Model file for the job. Use its own axes, mm. A direction names the side the tool comes from. Coordinates: 2 decimals unless noted, no trailing zeros. Write each loop counter-clockwise with the first axis right and the second up, starting at its lowest first coordinate (ties: lowest second). Pieces come first, ordered by that corner, then holes. Notation, with made-up numbers: (2.25, 48) -> (60.25, 48) arc R15 ccw to (60.25, 75) -> close; hole circle Ø5 at (81, 55). An arc over 180 degrees is marked (long way). Write item = value, one per line. Start each with the question number.
from build123d import *

# Parameters (mm, degrees)
SKETCH1_R           = 6
BOSS_EXTRUDE1_DEPTH = 4
SKETCH2_R           = 3
BOSS_EXTRUDE2_DEPTH = 4
SKETCH3_R           = 1.6
CUT_EXTRUDE1_DEPTH  = 16
CHAMFER1_SIZE       = 3


with BuildPart() as part:
    # Sketch1 → Boss-Extrude1 (new, symmetric)
    with BuildSketch(Plane(origin=(0, 0, 0), x_dir=(1, 0, 0), z_dir=(0, 1, 0))):
        with Locations(Location((0, 0, 0), (0, 0, 270))):
            Circle(SKETCH1_R)
    extrude(amount=BOSS_EXTRUDE1_DEPTH, both=True)

    # Sketch2 → Boss-Extrude2 (add)
    with BuildSketch(Plane(origin=(0, 4, 0), x_dir=(1, 0, 0), z_dir=(0, 1, 0))):
        with Locations(Location((0, 0, 0), (0, 0, 270))):
            Circle(SKETCH2_R)
    boss_extrude2 = extrude(amount=BOSS_EXTRUDE2_DEPTH)

    # Mirror1: Boss-Extrude2 across plane
    add(boss_extrude2.mirror(Plane.ZX))

    # Sketch3 → Cut-Extrude1 (cut)
    with BuildSketch(Plane(origin=(0, 8, 0), x_dir=(1, 0, 0), z_dir=(0, 1, 0))):
        with Locations(Location((0, 0, 0), (0, 0, 270))):
            Circle(SKETCH3_R)
    extrude(amount=-CUT_EXTRUDE1_DEPTH, mode=Mode.SUBTRACT)

    # Chamfer1
    chamfer1_edges = [part.edges().sort_by_distance(p)[0] for p in [
        (0, -4, -3),
        (0, 4, -3),
    ]]
    chamfer(chamfer1_edges, length=CHAMFER1_SIZE - 0.0001)  # a hair under: the kernel refuses the full size


solid = part.part
(1) Drop flat-ended pins along their axis: pin 1 Ø2 at (x, y) = (-4, -2.5) entering from -Z; pin 2 Ø1 at (x, z) = (-4.5, -3) entering from -Y; pin 3 Ø1.5 at (x, z) = (-4, -4) entering from +Y. Give the stop position or say it passes through.
(2) Mould opens along Z. For faces 1 (the face through (-1.3, 8, 1.3)), 2 (the face through (3.119, 6.854, -0.41)), 3 (the face through (-0.97, 0.11, -1.27)) say: released by +Z, released by -Z, zero draft, split by the parting line, or undercut.
(3) Saw through at C-C (y = 1). Give the cut face in (x, z), then the cut area to 3 significant figures.
(4) Saw through at D-D (y = -5.5). Give the cut face in (x, z).
(5) Drill centre lines: line 1 along X through (y, z) = (-1.25, 0); line 2 along Z through (x, y) = (-1.25, -3); line 3 along X through (y, z) = (-4.5, 0). Where is each one in solid material? Low to high.
(6) 3-axis set-ups, long thin cutter, end or side, ignore diameter. For faces 4 (the face through (0.9, 7.49, 2.86)), 5 (the face through (0.9, -7.49, 2.86)), 6 (the face through (1.802, 0.056, 5.723)): which of +Z, -Z, +X, -X, +Y, -Y reach the whole face in a straight line?
Returned:
q1.pin_1 = -5.2
q1.pin_2 = -5.09
q1.pin_3 = 5.09
q2.face_1 = zero draft
q2.face_2 = split by the parting line
q2.face_3 = undercut
q3.outline = circle Ø12 at (0, 0); hole circle Ø3.2 at (0, 0)
q3.area = 105 mm2
q4.outline = circle Ø9 at (0, 0); hole circle Ø3.2 at (0, 0)
q5.line_1 = -6 to -1.6, 1.6 to 6
q5.line_2 = -5.87 to -1, 1 to 5.87
q5.line_3 = -5.5 to -1.6, 1.6 to 5.5
q6.face_4 = +Y
q6.face_5 = -Y
q6.face_6 = +Y, -Y
